Part print with two shaded views. Sizes in mm from the minimum x, y, z corner. A direction names the side the tool comes from. Give positions to 0.01 mm unless a question says otherwise; leave off trailing zeros. Write each loop counter-clockwise with the first axis right and the second up, starting at its lowest first coordinate (ties: lowest second). Pieces come first, ordered by that corner, then holes. Notation, with made-up numbers: (23, 70) -> (29, 70) arc R22 ccw to (29, 88) -> close; hole circle Ø7 at (71.25, 43). An arc over 180 degrees is marked (long way). Use one line per item in the form item = value. Start each with the question number.
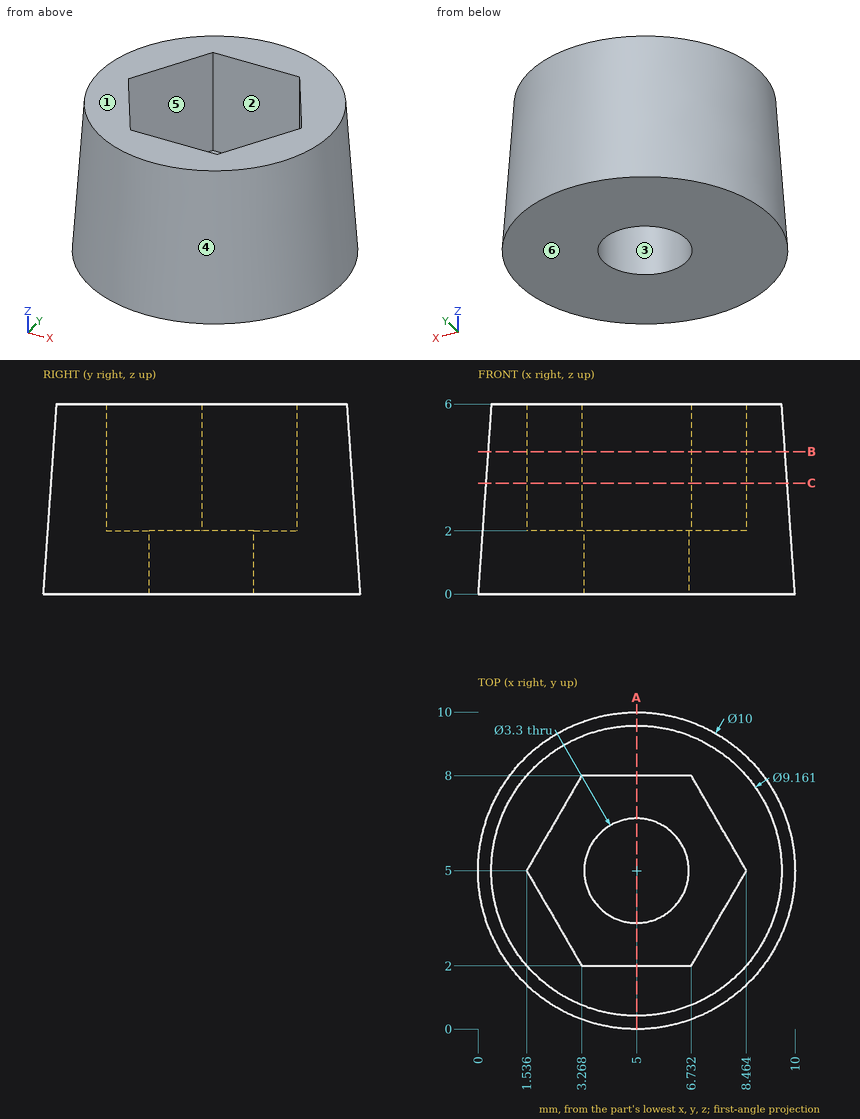
1) Cut at B-B (z = 4.5). Give the cut face in (x, y), and give its area (3 significant figures).
2) Two-plate mould, pull along X, no slides. Class the marked faces 3, 4, 5 and 6: released by +X, released by -X, zero draft, split by the parting line, or undercut.
3) Cut at C-C (z = 3.5). Give the cut face in (x, y).
4) 3-axis set-ups, long thin cutter, end or side, ignore diameter. For the marked faces 1 and 2: which of +Z, -Z, +X, -X, +Y, -Y reach the whole face in a straight line?
5) Pin check, flat tips, straight feed: pin 1 (3 mm diameter, centred on x = 4, y = 2.5, fed in from +Z); pin 2 (1.5 mm diameter, centred on x = 4.5, y = 5, fed in from +Z); pin 3 (1 mm diameter, centred on x = 7, z = 1.5, fed in from -Y); pin 4 (1 mm diameter, centred on x = 5, z = 4.5, fed in from +Y). Stop position of each tip, or through.
6) Cut at A-A (x = 5). Give the cut face in (y, z), and give its area (3 significant figures).
7) Wall check: line 1 along X through (y, z) = (4.75, 1.5); line 2 along Y through (x, z) = (7, 4.75) (1 decimal); line 3 along Z through (x, y) = (2.5, 6.25). Give the ranges that are in metal, low to high. Write a range as from..to.
Final values:
q1.outline = circle Ø9.37 at (5, 5); hole (1.54, 5) -> (3.27, 2) -> (6.73, 2) -> (8.46, 5) -> (6.73, 8) -> (3.27, 8) -> close
q1.area = 37.8 mm^2
q2.face_3 = undercut
q2.face_4 = split by the parting line
q2.face_5 = undercut
q2.face_6 = zero draft
q3.outline = circle Ø9.51 at (5, 5); hole (1.54, 5) -> (3.27, 2) -> (6.73, 2) -> (8.46, 5) -> (6.73, 8) -> (3.27, 8) -> close
q4.face_1 = +Z, +X, -X, +Y, -Y
q4.face_2 = +Z
q5.pin_1 = 6
q5.pin_2 = through
q5.pin_3 = 0.34
q5.pin_4 = 9.72
q6.outline = (0, 0) -> (3.35, 0) -> (3.35, 2) -> (2, 2) -> (2, 6) -> (0.42, 6) -> close; (6.65, 0) -> (10, 0) -> (9.58, 6) -> (8, 6) -> (8, 2) -> (6.65, 2) -> close
q6.area = 26.9 mm^2
q7.line_1 = 0.11..3.37, 6.63..9.89
q7.line_2 = 0.8..2.5, 7.5..9.2
q7.line_3 = 0..2
